Geometry: final body of the model. Coordinates: model frame, mm. A direction names the side the tool comes from. Coordinates: 2 decimals unless noted, no trailing zeros. Order: outer loops, then holes, each group sorted by start corner. A loop starts at its lowest first (then second) coordinate and runs counter-clockwise, first axis right, second up. Notation, with made-up numbers: (-19, 43.5) -> (31, 43.5) arc R19 cw to (31, 79.5) -> close; hole circle Ø8 at (69.25, 79). An arc over 180 degrees is marked (long way). Answer in a Markdown table with one row per item. Add a question column.
1) Pull-direction query (Z, two-part tool) for faces 1 (the face through (10, 10, -2)), 2 (the face through (10, -10, -2)), 3 (the face through (32, 0, -12.5)), 4 (the face through (-9, -35, 3)); classes: +Z half, -Z half, draft (parallel to the pull), parting line (faces both ways), or undercut.
2) Section query A-A on x = -28. Return the cut outline in (y, z).
3) Section query B-B on y = 19.5. Return the cut outline in (x, z).
4) Section query D-D on x = 15. Return the cut outline in (y, z).
5) Section query C-C on y = 4. Return the cut outline in (x, z).
6) Contact query for flat-ended pins moving along their axis: P1, Ø1.5, axis at y = -4, z = 2, coming from the -X side; P2, Ø6, axis at x = 3, z = 2, coming from the +Y side; P3, Ø6, axis at x = 26.5, y = -5.5, coming from the -Z side. Output: stop coordinate, or through.
7) Set-up query: faces 5 (the face through (24.153, -22.325, 1.343)), 6 (the face through (-28, 15, 0)), 7 (the face through (-38, -10, 0)), 8 (the face through (-19.7, 0.5, -12.5)), 9 (the face through (-3.844, 22.675, 1.651)). Return all of +Z, -Z, +X, -X, +Y, -Y with unobstructed straight access to the full face (end or side cutting, diameter ignored); none if empty.
8) Ray query, line 1 (Y direction, x = -28, z = 9); line 2 (X direction, y = -14.5, z = 6); line 3 (X direction, y = 13.5, z = 3.5). Return the intervals inside material, ascending. Write a range as from..to.
```python
from build123d import *

# Parameters (mm, degrees)
F0_W          = 70
F0_H          = 25
F1_DEPTH      = 40
F1_DEPTH_BACK = 40
F3_DEPTH      = 40
F4_W          = 40
F4_H          = 20
F5_DEPTH      = 25
F7_DEPTH      = 25
F8_W          = 80
F8_H          = 25
F9_DEPTH      = 35
F11_DEPTH     = 25
F12_T4_DEPTH  = 76.2347538298
F12_T9_DEPTH  = 76.2347538298
F12_T14_DEPTH = 76.2347538298
F12_T19_DEPTH = 76.2347538298


# Not quite as in the source:
# - a fillet or chamfer that OpenCascade refuses, or shapes differently, is made with other operations: its cross-section is extruded or revolved along the edge and cut away or added


with BuildPart() as f1:
    # F0 (on Right) → F1 (new body, two sides)
    with BuildSketch(Plane.YZ) as f1_sk:
        Rectangle(F0_W, F0_H)
    extrude(amount=F1_DEPTH)
    extrude(f1_sk.sketch, amount=-F1_DEPTH_BACK)

    # F2 (on face) → F3 (cut)
    with BuildSketch(Plane.XY.offset(12.5)):
        Polygon((-40, 10), (-40, 0), (-20, 0), (-20, 15), (-35, 15), (-35, 10), align=None)
        Polygon((-20, 0), (-40, 0), (-40, -10), (-35, -10), (-35, -15), (-20, -15), align=None)
    extrude(amount=-F3_DEPTH, mode=Mode.SUBTRACT)

    # F4 (on face) → F5 (cut)
    with BuildSketch(Plane.XZ.offset(35)):
        with Locations((10, -2.5)):
            Rectangle(F4_W, F4_H)
    extrude(amount=-F5_DEPTH, mode=Mode.SUBTRACT)

    # F6 (on face) → F7 (join)
    with BuildSketch(Plane.XZ.offset(10)):
        with BuildLine():
            Line((0, -12.5), (20, -12.5))
            ThreePointArc((20, -12.5), (10, -2.5), (0, -12.5))
        make_face()
        with BuildLine():
            ThreePointArc((0, -12.5), (10, -22.5), (20, -12.5))
            Line((20, -12.5), (0, -12.5))
        make_face()
    extrude(amount=F7_DEPTH)

    # F8 (on face) → F9 (cut)
    with BuildSketch(Plane(origin=(0, 35, 0), x_dir=(-1, 0, 0), z_dir=(0, 1, 0))):
        Rectangle(F8_W, F8_H)
    extrude(amount=-F9_DEPTH, mode=Mode.SUBTRACT)

    # F10: F1 across plane


with BuildPart() as f1_1:
    add(f1.part)
    add(f1.part.mirror(Plane.XZ))

    # F11 (add): a face of the model
    f11_faces = [f1_1.faces().sort_by_distance(p)[0] for p in [
        (10, -10, -16.7441318158),
    ]]
    extrude(f11_faces, amount=F11_DEPTH)

    # F12: fillet of radius 20.5 on 4 edges, made by hand


with BuildPart() as f12_tool2:
    # F12_s3 → F12_t4 (new body)
    with BuildSketch(Plane.XZ.offset(-35)):
        with BuildLine():
            ThreePointArc((30, -12.5), (23.8239195314, 1.6714007511), (9.5060984681, 7.5))
            Line((9.5060984681, 7.5), (30, 7.5))
            Line((30, 7.5), (30, -12.5))
        make_face()
    extrude(amount=F12_T4_DEPTH)

    split(bisect_by=Plane.XZ.offset(35), keep=Keep.BOTTOM)


with BuildPart() as f1_2:
    add(f1_1.part)

    # F12_t1: union F12_tool2
    add(f12_tool2.part)


with BuildPart() as f12_tool7:
    # F12_s8 → F12_t9 (new body)
    with BuildSketch(Plane.XZ.offset(-35)):
        with BuildLine():
            ThreePointArc((10.4939015319, 7.5), (-3.8239195314, 1.6714007511), (-10, -12.5))
            Line((-10, -12.5), (-10, 7.5))
            Line((-10, 7.5), (10.4939015319, 7.5))
        make_face()
    extrude(amount=F12_T9_DEPTH)

    split(bisect_by=Plane.XZ.offset(35), keep=Keep.BOTTOM)


with BuildPart() as f1_3:
    add(f1_2.part)

    # F12_t6: union F12_tool7
    add(f12_tool7.part)


with BuildPart() as f12_tool12:
    # F12_s13 → F12_t14 (new body)
    with BuildSketch(Plane.XZ.offset(35)):
        with BuildLine():
            ThreePointArc((30, -12.5), (23.8239195314, 1.6714007511), (9.5060984681, 7.5))
            Line((9.5060984681, 7.5), (30, 7.5))
            Line((30, 7.5), (30, -12.5))
        make_face()
    extrude(amount=-F12_T14_DEPTH)

    split(bisect_by=Plane.XZ.offset(-35), keep=Keep.TOP)


with BuildPart() as f1_4:
    add(f1_3.part)

    # F12_t11: union F12_tool12
    add(f12_tool12.part)


with BuildPart() as f12_tool17:
    # F12_s18 → F12_t19 (new body)
    with BuildSketch(Plane.XZ.offset(35)):
        with BuildLine():
            ThreePointArc((-10, -12.5), (-3.8239195314, 1.6714007511), (10.4939015319, 7.5))
            Line((10.4939015319, 7.5), (-10, 7.5))
            Line((-10, 7.5), (-10, -12.5))
        make_face()
    extrude(amount=-F12_T19_DEPTH)

    split(bisect_by=Plane.XZ.offset(-35), keep=Keep.TOP)


with BuildPart() as f1_5:
    add(f1_4.part)

    # F12_t16: union F12_tool17
    add(f12_tool17.part)


solid = f1_5.part
```
Result:
| question | item | result |
|---|---|---|
| 1 | face 1 | undercut |
| 1 | face 2 | undercut |
| 1 | face 3 | -Z half |
| 1 | face 4 | draft |
| 2 | outline | (-35, -12.5) -> (-15, -12.5) -> (-15, 12.5) -> (-35, 12.5) -> close; (15, -12.5) -> (35, -12.5) -> (35, 12.5) -> (15, 12.5) -> close |
| 3 | outline | (-40, -12.5) -> (-10, -12.5) arc R20.5 cw to (10, 7.49) arc R20.5 cw to (30, -12.5) -> (40, -12.5) -> (40, 12.5) -> (-40, 12.5) -> close; circle Ø20 at (10, -12.5) |
| 4 | outline | (-35, -21.16) -> (35, -21.16) -> (35, -3.84) -> (10, -3.84) -> (10, 6.75) -> (35, 6.75) -> (35, 12.5) -> (-35, 12.5) -> (-35, 6.75) -> (-10, 6.75) -> (-10, -3.84) -> (-35, -3.84) -> close |
| 5 | outline | (-20, -12.5) -> (0, -12.5) arc R10 ccw to (20, -12.5) -> (40, -12.5) -> (40, 12.5) -> (-20, 12.5) -> close |
| 6 | P1 | x = -20 |
| 6 | P2 | y = 10 |
| 6 | P3 | z = -12.5 |
| 7 | face 5 | -Y |
| 7 | face 6 | +Z, -Z |
| 7 | face 7 | +Z, -Z, -X |
| 7 | face 8 | -Z, -X, +Y, -Y |
| 7 | face 9 | +Y |
| 8 | line 1 | -35..-15, 15..35 |
| 8 | line 2 | -40..-35, -20..2.8, 17.2..40 |
| 8 | line 3 | -40..-35, -20..-1.67, 21.67..40 |
